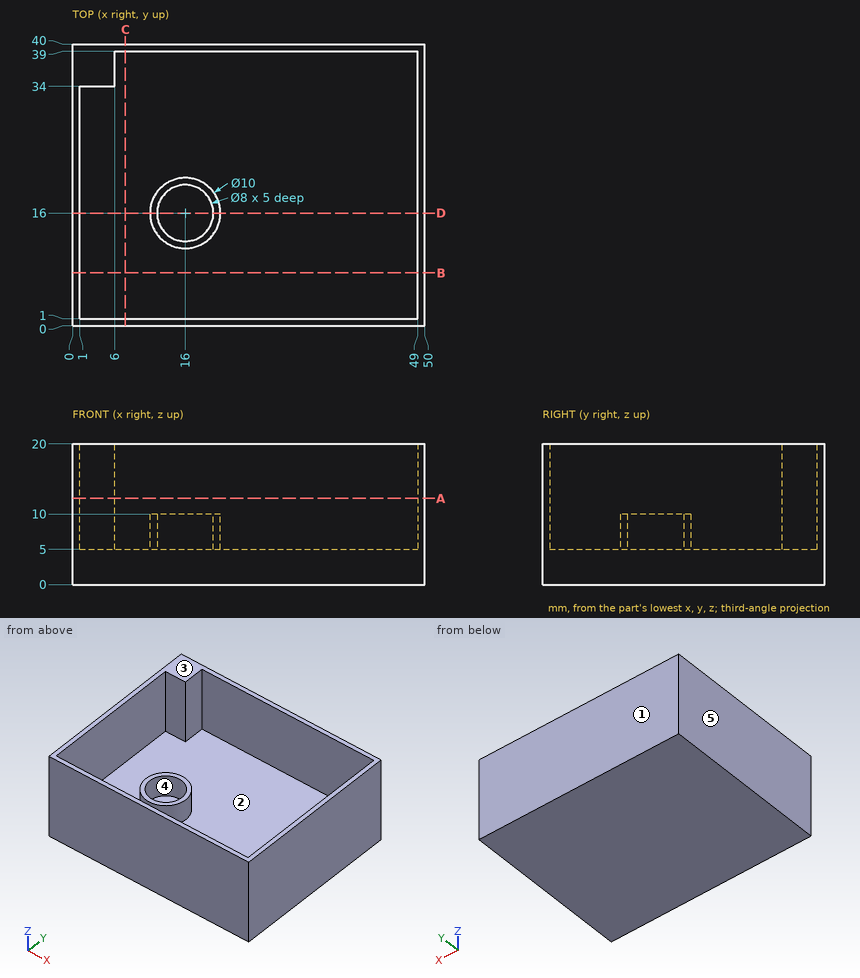
The drawing under review shows one solid part. Ordinate dimensions are in mm from its lowest x, y, z. A direction names the side the tool comes from. Round coordinates to 2 decimals unless told otherwise and drop trailing zeros. Loops run counter-clockwise (first coordinate to the right, second up) from the corner with the lowest first, then second, coordinate; pieces in that order, holes last. Notation, with made-up numbers: (57, 4) -> (62, 4) arc R19 ccw to (62, 20) -> close; hole circle Ø8 at (67, -14.75). An arc over 180 degrees is marked (long way). One line per question, with ' | ' between items. Start each with the question number.
Item 1: Add section A-A, the plane z = 12.25. Write out the cut boundary in (x, y).
Item 2: Add section D-D, the plane y = 16. Write out the cut boundary in (x, z).
Item 3: Add section C-C, the plane x = 7.5. Write out the cut boundary in (y, z).
Item 4: Machinability: for the marked faces 4 and 5, which of the approach directions +Z, -Z, +X, -X, +Y, -Y give a long, thin tool a straight path to every point of the face, cutting with its end or side? Answer none if there is none.
Item 5: For pin 1 (9 mm diameter, centred on x = 15.5, y = 17, fed in from +Z), flat-tipped, find the tip position at first contact; note if it passes through.
Item 6: Wall thickness on line 1 along Y through (x, z) = (16, 8.2); line 2 along X through (y, z) = (3, 11.5); line 3 along Y through (x, z) = (7, 6.25): over which ranges is each line inside the solid? List them lowest first. Write a range as [from, to].
Item 7: Draft analysis for pull direction Y (two halves, no side actions). For the marked faces 1, 2 and 3, state which applies: +Y half, -Y half, draft (parallel to the pull), parting line (faces both ways), or undercut.
Item 8: Add section B-B, the plane y = 7.5. Write out the cut boundary in (x, z).
Return value:
1) outline: (0, 0) -> (50, 0) -> (50, 40) -> (0, 40) -> close; hole (1, 1) -> (49, 1) -> (49, 39) -> (6, 39) -> (6, 34) -> (1, 34) -> close
2) outline: (0, 0) -> (50, 0) -> (50, 20) -> (49, 20) -> (49, 5) -> (21, 5) -> (21, 10) -> (20, 10) -> (20, 5) -> (12, 5) -> (12, 10) -> (11, 10) -> (11, 5) -> (1, 5) -> (1, 20) -> (0, 20) -> close
3) outline: (0, 0) -> (40, 0) -> (40, 20) -> (39, 20) -> (39, 5) -> (1, 5) -> (1, 20) -> (0, 20) -> close
4) face 4: +Z | face 5: +Z, -Z, -X, +Y, -Y
5) pin 1: stops at z = 10
6) line 1: y = [0, 1], [11, 12], [20, 21], [39, 40] | line 2: x = [0, 1], [49, 50] | line 3: y = [0, 1], [39, 40]
7) face 1: +Y half | face 2: undercut | face 3: draft
8) outline: (0, 0) -> (50, 0) -> (50, 20) -> (49, 20) -> (49, 5) -> (1, 5) -> (1, 20) -> (0, 20) -> close
